Build history of the part. All positions in model axes, mm. A direction names the side the tool comes from. Give positions to 0.01 mm unless a question says otherwise; leave off trailing zeros. Order: outer loops, then holes, each group sorted by start corner. A loop starts at its lowest first (then second) coordinate and runs counter-clockwise, first axis right, second up. Notation, with made-up numbers: M 64.5,-16 L 119.5,-16 A29 cw 119.5,4 Z; hole C -14.5,35.5 d4. An arc over 180 degrees is marked long. One line per item, written item: value.
from build123d import *

# Parameters (mm, degrees)
CROQUIS1_R              = 7
SALIENTE_EXTRUIR1_DEPTH = 38.1
SALIENTE_EXTRUIR2_DEPTH = 11
CROQUIS3_R              = 27.5
CROQUIS3_R_2            = 10
CORTAR_EXTRUIR1_DEPTH   = 8
CORTAR_EXTRUIR1_DRAFT   = -48
CROQUIS4_R              = 37.959799744
CROQUIS4_R_2            = 10.5
CORTAR_EXTRUIR2_DEPTH   = 11
CORTAR_EXTRUIR2_DRAFT   = -48


with BuildPart() as part:
    # Croquis1 → Saliente-Extruir1 (new body)
    with BuildSketch(Plane.XY):
        with Locations(Location((0, 0, 0), (0, 0, 180))):
            Circle(CROQUIS1_R)
    extrude(amount=SALIENTE_EXTRUIR1_DEPTH)

    # Croquis2 → Saliente-Extruir2 (add)
    with BuildSketch(Plane.XY.offset(38.1)):
        Polygon((12.124355653, 0), (6.062177826, 10.5), (-6.062177826, 10.5), (-12.124355653, 0), (-6.062177826, -10.5), (6.062177826, -10.5), align=None)
    extrude(amount=SALIENTE_EXTRUIR2_DEPTH)


with BuildPart() as cortar_extruir1_tool:
    # Croquis3 → Cortar-Extruir1 (with draft: the straight prism first)
    with BuildSketch(Plane.XY.offset(49.1)):
        Circle(CROQUIS3_R)
        Circle(CROQUIS3_R_2, mode=Mode.SUBTRACT)
    extrude(amount=-CORTAR_EXTRUIR1_DEPTH)
    # Cortar-Extruir1: the draft: its side faces are tilted about the plane it starts from
    cortar_extruir1_sides = [cortar_extruir1_tool.faces().sort_by_distance(p)[0] for p in [
        (-27.5, 0, 45.1),
        (-10, 0, 45.1),
    ]]
    draft(cortar_extruir1_sides, Plane.XY.offset(49.1), CORTAR_EXTRUIR1_DRAFT)


with BuildPart() as part_1:
    add(part.part)

    # Cortar-Extruir1: cut by cortar_extruir1_tool
    add(cortar_extruir1_tool.part, mode=Mode.SUBTRACT)


with BuildPart() as cortar_extruir2_tool:
    # Croquis4 → Cortar-Extruir2 (with draft: the straight prism first)
    with BuildSketch(Plane(origin=(0, 0, 38.1), x_dir=(-1, 0, 0), z_dir=(0, 0, -1))):
        Circle(CROQUIS4_R)
        Circle(CROQUIS4_R_2, mode=Mode.SUBTRACT)
    extrude(amount=-CORTAR_EXTRUIR2_DEPTH)
    # Cortar-Extruir2: the draft: its side faces are tilted about the plane it starts from
    cortar_extruir2_sides = [cortar_extruir2_tool.faces().sort_by_distance(p)[0] for p in [
        (37.959799744, 0, 43.6),
        (10.5, 0, 43.6),
    ]]
    draft(cortar_extruir2_sides, Plane(origin=(0, 0, 38.1), x_dir=(-1, 0, 0), z_dir=(0, 0, -1)), CORTAR_EXTRUIR2_DRAFT)


with BuildPart() as part_2:
    add(part_1.part)

    # Cortar-Extruir2: cut by cortar_extruir2_tool
    add(cortar_extruir2_tool.part, mode=Mode.SUBTRACT)


solid = part_2.part
1) Tool access for faces 1 (the face through (-6.466, 2.681, 18.783)), 2 (the face through (5.467, -9.415, 38.449)): list every direction of +Z, -Z, +X, -X, +Y, -Y with a clear straight run to the whole face (end or side of a thin tool).
Check values:
face 1: -Z
face 2: -Z, +X, -Y
2) Drill centre lines: probe 1 along X at (y, z) = (0.25, 24); probe 2 along X at (y, z) = (-5.25, 46.5); probe 3 along Z at (x, y) = (9.25, 0.75). Where is each one in solid material? Low to high. Write a range as from..to.
Check values:
probe 1: -7..7
probe 2: -9.09..9.09
probe 3: 38.1..49.1
3) Saw through at A-A, the plane z = 12. Write the cut outline in (x, y).
Check values:
outline: C 0,0 d14
4) Pin check, flat tips, straight feed: pin 1 (1 mm diameter, centred on x = 8, z = 23, fed in from -Y); pin 2 (1.5 mm diameter, centred on x = 3, z = 35.5, fed in from -Y); pin 3 (6 mm diameter, centred on x = -4, z = 19, fed in from -Y); pin 4 (4 mm diameter, centred on x = 4.5, z = 30, fed in from +Y). Stop position of each tip, or through.
Check values:
pin 1: through
pin 2: y = -6.63
pin 3: y = -6.93
pin 4: y = 6.54
